Check sheet for the modelled part. Datum: model origin and axes. Units: mm. A direction names the side the tool comes from. Round coordinates to 2 decimals unless told otherwise and drop trailing zeros. Order: outer loops, then holes, each group sorted by start corner. A loop starts at its lowest first (then second) coordinate and runs counter-clockwise, first axis right, second up. Notation, with made-up numbers: M 64.5,46 L 83.5,46 A21 cw 83.5,68 Z; hole C 16,-16.5 d6. An arc over 180 degrees is marked long. One line per item, written item: value. Start each with the question number.
(1) Depth check by flat-ended pin: pin 1 Ø6.5 at (x, z) = (-1, -37) entering from -Y; pin 2 Ø1 at (x, z) = (2.5, -47) entering from -Y; pin 3 Ø3 at (y, z) = (-0.5, -28.5) entering from +X. Enter the tip coordinate at first touch or a pass-through.
(2) Thickness scan on L1, parallel to Y at x = 0, z = -77.5; L2, parallel to Y at x = -6.75, z = -95; L3, parallel to X at y = 5, z = -7.5. Record the ranges inside material, lowest first.
(3) Release check for a two-part mould opening along Y. For faces 1 (the face through (-5.11, -4.26, -49.3)), 2 (the face through (2, -2, 0)), 3 (the face through (9.395, 9.362, -49.3)) record: released by +Y, released by -Y, zero draft, split by the parting line, or undercut.
(4) Access from +Z, -Z, +X, -X, +Y, -Y to the whole of each face (thin tool, end or side, straight path). Record for faces 4 (the face through (-9.211, 3.354, -49.3)), 5 (the face through (-3.354, -9.211, -49.3)), 6 (the face through (-5.5, 7, -49)), 7 (the face through (-3.347, 9.189, -49.3)).
(5) Cross-section at A-A, the plane x = 0. Enter the section's corners in (y, z).
from build123d import *

# Parameters (mm, degrees)
SKETCH_1_R      = 2.5
EXTRUDE_1_DEPTH = 100


with BuildPart() as part:
    # 草图1 → 凸台-拉伸1 (new body)
    with BuildSketch(Plane.XY):
        with BuildLine():
            ThreePointArc((-7.878679656, 10), (-9.378679656, 9.378679656), (-10, 7.878679656))
            Line((-10, 7.878679656), (-10, 3.6))
            Line((-10, 3.6), (-8.4, 3.1))
            Line((-8.4, 3.1), (-8.4, 5.5))
            Line((-8.4, 5.5), (-6.348528137, 5.5))
            Line((-6.348528137, 5.5), (-3.9, 3.051471863))
            Line((-3.9, 3.051471863), (-3.9, -3.051471863))
            Line((-3.9, -3.051471863), (-6.348528137, -5.5))
            Line((-6.348528137, -5.5), (-8.4, -5.5))
            Line((-8.4, -5.5), (-8.4, -3.1))
            Line((-8.4, -3.1), (-10, -3.6))
            Line((-10, -3.6), (-10, -7.878679656))
            ThreePointArc((-10, -7.878679656), (-9.378679656, -9.378679656), (-7.878679656, -10))
            Line((-7.878679656, -10), (-3.6, -10))
            Line((-3.6, -10), (-3.1, -8.4))
            Line((-3.1, -8.4), (-5.5, -8.4))
            Line((-5.5, -8.4), (-5.5, -6.348528137))
            Line((-5.5, -6.348528137), (-3.051471863, -3.9))
            Line((-3.051471863, -3.9), (3.051471863, -3.9))
            Line((3.051471863, -3.9), (5.5, -6.348528137))
            Line((5.5, -6.348528137), (5.5, -8.4))
            Line((5.5, -8.4), (3.1, -8.4))
            Line((3.1, -8.4), (3.6, -10))
            Line((3.6, -10), (7.878679656, -10))
            ThreePointArc((7.878679656, -10), (9.378679656, -9.378679656), (10, -7.878679656))
            Line((10, -7.878679656), (10, -3.6))
            Line((10, -3.6), (8.4, -3.1))
            Line((8.4, -3.1), (8.4, -5.5))
            Line((8.4, -5.5), (6.348528137, -5.5))
            Line((6.348528137, -5.5), (3.9, -3.051471863))
            Line((3.9, -3.051471863), (3.9, 3.051471863))
            Line((3.9, 3.051471863), (6.348528137, 5.5))
            Line((6.348528137, 5.5), (8.4, 5.5))
            Line((8.4, 5.5), (8.4, 3.1))
            Line((8.4, 3.1), (10, 3.6))
            Line((10, 3.6), (10, 7.878679656))
            ThreePointArc((10, 7.878679656), (9.378679656, 9.378679656), (7.878679656, 10))
            Line((7.878679656, 10), (6.359631643, 10))
            Line((6.359631643, 10), (3.6, 10))
            Line((3.6, 10), (3.1, 8.4))
            Line((3.1, 8.4), (5.5, 8.4))
            Line((5.5, 8.4), (5.5, 6.348528137))
            Line((5.5, 6.348528137), (3.051471863, 3.9))
            Line((3.051471863, 3.9), (-3.051471863, 3.9))
            Line((-3.051471863, 3.9), (-5.5, 6.348528137))
            Line((-5.5, 6.348528137), (-5.5, 8.4))
            Line((-5.5, 8.4), (-3.1, 8.4))
            Line((-3.1, 8.4), (-3.6, 10))
            Line((-3.6, 10), (-6.359631643, 10))
            Line((-6.359631643, 10), (-7.878679656, 10))
        make_face()
        Circle(SKETCH_1_R, mode=Mode.SUBTRACT)
    extrude(amount=-EXTRUDE_1_DEPTH)


solid = part.part
Values found:
1. pin 1: y = -10
1. pin 2: y = -3.9
1. pin 3: x = 3.9
2. L1: -3.9 to -2.5, 2.5 to 3.9
2. L2: -10 to -5.5, 5.5 to 10
2. L3: -10 to -8.4, -5.85 to -4.15, 4.15 to 5.85, 8.4 to 10
3. face 1: undercut
3. face 2: zero draft
3. face 3: released by +Y
4. face 4: +Z, -Z, -X
4. face 5: +Z, -Z, -Y
4. face 6: +Z, -Z
4. face 7: +Z, -Z, +Y
5. outline: M -3.9,-100 L -2.5,-100 L -2.5,0 L -3.9,0 Z; M 2.5,-100 L 3.9,-100 L 3.9,0 L 2.5,0 Z
